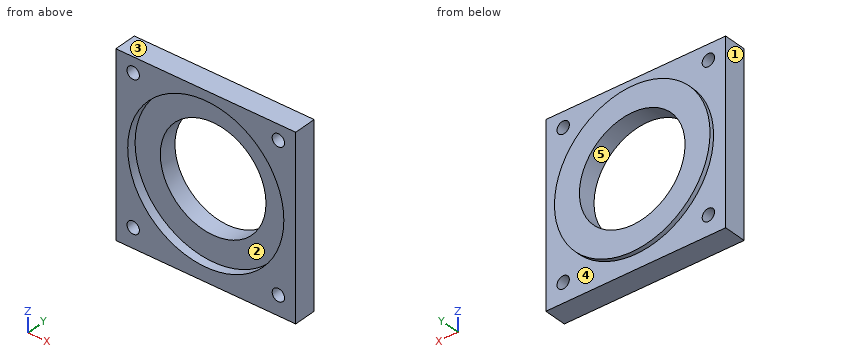
```python
from build123d import *

# Parameters (mm, degrees)
F0_W     = 127
F0_H     = 127
F2_DEPTH = 15.875
F3_R     = 37.2999
F4_DEPTH = 16.002
F5_R     = 55.118
F5_R_2   = 37.2999
F6_DEPTH = 6.35
F7_R     = 54.9275
F7_R_2   = 37.2999
F8_DEPTH = 3.048
F10_D    = 8.73125


# Not quite as in the source:
# - a length typed as a fraction of an inch, garbled in the dataset ("3 / 203.2 mm" for 3/8 in), is restored


with BuildPart() as f2:
    # F0 (on Front) → F2 (new body)
    with BuildSketch(Plane.XZ):
        with Locations((-63.5, 63.5)):
            Rectangle(F0_W, F0_H)
    extrude(amount=F2_DEPTH)

    # F3 (on face) → F4 (cut)
    with BuildSketch(Plane.XZ.offset(15.875)):
        with Locations((-63.5, 65.0875)):
            Circle(F3_R)
    extrude(amount=-F4_DEPTH, mode=Mode.SUBTRACT)

    # F5 (on face) → F6 (cut)
    with BuildSketch(Plane.XZ.offset(15.875)):
        with Locations((-63.5, 65.0875)):
            Circle(F5_R)
        with Locations((-63.5, 65.0875)):
            Circle(F5_R_2, mode=Mode.SUBTRACT)
    extrude(amount=-F6_DEPTH, mode=Mode.SUBTRACT)

    # F7 (on face) → F8 (join)
    with BuildSketch(Plane.XZ):
        with Locations((-63.5, 65.0875)):
            Circle(F7_R)
        with Locations((-63.5, 65.0875)):
            Circle(F7_R_2, mode=Mode.SUBTRACT)
    extrude(amount=-F8_DEPTH)

    # F10 (through all)
    with Locations(Plane.XZ.offset(15.875)):
        with Locations((-114.7572, 116.3447), (-12.2428, 116.3447), (-12.2428, 13.8303), (-114.7572, 13.8303)):
            Hole(F10_D / 2)


solid = f2.part
```
Source: CAD feature listing. Evaluate the final solid. Frame: model axes, mm. Face numbers are marked on the shaded views. A direction names the side the tool comes from. Round coordinates to 2 decimals unless told otherwise and drop trailing zeros. Order: outer loops, then holes, each group sorted by start corner. A loop starts at its lowest first (then second) coordinate and runs counter-clockwise, first axis right, second up. Notation, with made-up numbers: (58.25, 88.25) -> (99.25, 88.25) arc R27 cw to (99.25, 118.25) -> close; hole circle Ø3 at (32, -21.5). An arc over 180 degrees is marked (long way). One line per item, written item: value. Start each with the question number.
Q1. Section query B-B (y = -13.25). Return the cut outline in (x, z).
Q2. Pin query (flat end, axial travel): pin 1 (10 mm diameter, centred on x = -12.24, z = 116.34, fed in from +Y); pin 2 (1 mm diameter, centred on x = -42, z = 99.5, fed in from -Y) (3 decimals); pin 3 (1.5 mm diameter, centred on x = -41.5, y = 1, fed in from -Z). Return the tip coordinate at first contact, or that it passes through.
Q3. Section query C-C (z = 29.5). Return the cut outline in (x, y) (3 decimals).
Q4. Material intervals for probe 1 along Z at (x, y) = (-63.5, -13); probe 2 along Z at (x, y) = (-113, -3.5); probe 3 along X at (y, z) = (-12.5, 114), sorted ascending.
Q5. Access query for the marked faces 4 and 5. Directions: +Z, -Z, +X, -X, +Y, -Y. A direction counts if a zero-diameter tool reaches every point of the face in a straight line with its end or side. Return the directions, or none.
Q6. Section query A-A (x = -63.5). Return the cut outline in (y, z) (1 decimal), plus the area to 3 significant figures.
Q7. Section query D-D (x = -113). Return the cut outline in (y, z) (3 decimals).
Q8. Draft query along X for the marked faces 1, 2 and 3. Return one class per face: pulls with the +X half, pulls with the -X half, needs draft (parallel to the pull), parting line crosses it, or undercut.
Findings below:
1. outline: (-127, 0) -> (0, 0) -> (0, 127) -> (-127, 127) -> close; hole circle Ø8.73 at (-114.76, 13.83); hole circle Ø8.73 at (-114.76, 116.34); hole circle Ø110.24 at (-63.5, 65.09); hole circle Ø8.73 at (-12.24, 13.83); hole circle Ø8.73 at (-12.24, 116.34)
2. pin 1: y = 0
2. pin 2: y = -9.525
2. pin 3: z = 14.44
3. outline: (-127, -15.875) -> (-105.589, -15.875) -> (-105.589, -9.525) -> (-74.672, -9.525) -> (-74.672, 3.048) -> (-105.34, 3.048) -> (-105.34, 0) -> (-127, 0) -> close; (-52.328, -9.525) -> (-21.411, -9.525) -> (-21.411, -15.875) -> (0, -15.875) -> (0, 0) -> (-21.66, 0) -> (-21.66, 3.048) -> (-52.328, 3.048) -> close
4. probe 1: 0 to 9.97, 120.21 to 127
4. probe 2: 0 to 9.83, 17.83 to 112.35, 120.34 to 127
4. probe 3: -127 to -118.44, -111.07 to -88.91, -38.09 to -15.93, -8.56 to 0
5. face 4: +Y
5. face 5: +Y, -Y
6. outline: (-15.9, 0) -> (0, 0) -> (0, 10.2) -> (3, 10.2) -> (3, 27.8) -> (-9.5, 27.8) -> (-9.5, 10) -> (-15.9, 10) -> close; (-15.9, 120.2) -> (-9.5, 120.2) -> (-9.5, 102.4) -> (3, 102.4) -> (3, 120) -> (0, 120) -> (0, 127) -> (-15.9, 127) -> close
6. area: 713 mm²
7. outline: (-15.875, 0) -> (0, 0) -> (0, 9.834) -> (-15.875, 9.834) -> close; (-15.875, 17.827) -> (0, 17.827) -> (0, 41.28) -> (3.048, 41.28) -> (3.048, 88.895) -> (0, 88.895) -> (0, 112.348) -> (-15.875, 112.348) -> (-15.875, 89.331) -> (-9.525, 89.331) -> (-9.525, 40.844) -> (-15.875, 40.844) -> close; (-15.875, 120.341) -> (0, 120.341) -> (0, 127) -> (-15.875, 127) -> close
8. face 1: pulls with the -X half
8. face 2: undercut
8. face 3: needs draft
